from build123d import *

# Parameters (mm, degrees)
SKETCH1_W           = 76.2
SKETCH1_H           = 200.35
SKETCH1_R           = 19.05
SKETCH1_R_2         = 4.5
SKETCH1_R_3         = 3.25
BOSS_EXTRUDE1_DEPTH = 6.35


with BuildPart() as part:
    # Sketch1 → Boss-Extrude1 (new body)
    with BuildSketch(Plane.XY):
        with Locations((0, -25.175)):
            Rectangle(SKETCH1_W, SKETCH1_H)
        Circle(SKETCH1_R, mode=Mode.SUBTRACT)
        with Locations((0, 58.34)):
            Circle(SKETCH1_R_2, mode=Mode.SUBTRACT)
        with Locations((0, -58.34)):
            Circle(SKETCH1_R_2, mode=Mode.SUBTRACT)
        with Locations((-20, -110.35)):
            Circle(SKETCH1_R_3, mode=Mode.SUBTRACT)
        with Locations((20, -110.35)):
            Circle(SKETCH1_R_3, mode=Mode.SUBTRACT)
        with Locations((0, -77.35)):
            Circle(SKETCH1_R_3, mode=Mode.SUBTRACT)
    extrude(amount=BOSS_EXTRUDE1_DEPTH)


solid = part.part
Geometry: final body of the model. Coordinates: model frame, mm. Coordinates: 2 decimals unless noted, no trailing zeros. Loops run counter-clockwise (first coordinate to the right, second up) from the corner with the lowest first, then second, coordinate; pieces in that order, holes last. Notation, with made-up numbers: (71, -2.5) - (116, -2.5) arc R20 cw to (116, 29.5) - close; hole circle Ø6 at (62, 70). An arc over 180 degrees is marked (long way). One line per question, with ' | ' between items. Start each with the question number.
(1) Cut plane C-C on z = 3.25. Output: boundary loops of the cut face in (x, y).
(2) Ray query, L1, parallel to Y at x = 0, z = 4.5; L2, parallel to Y at x = -19.5, z = 1.75; L3, parallel to Y at x = 4, z = 3.5. Return the intervals inside material, ascending. Write a range as from..to.
(3) Cut plane B-B on x = 0. Output: boundary loops of the cut face in (y, z), and give its area (3 significant figures).
(4) Cut plane D-D on y = -110.35. Output: boundary loops of the cut face in (x, z).
(5) Draft query along Y for faces 1 (the flat face through (-1, -24, 6.35)), 2 (the cylindrical face through (-15.12, -11.59, 3.13)), 3 (the flat face through (-1, -125.35, 3)). Return one class per face: +Y half, -Y half, draft (parallel to the pull), parting line (faces both ways), or undercut.
(6) Cut plane A-A on y = -77.35. Output: boundary loops of the cut face in (x, z).
Here are the results:
1) outline: (-38.1, -125.35) - (38.1, -125.35) - (38.1, 75) - (-38.1, 75) - close; hole circle Ø6.5 at (-20, -110.35); hole circle Ø38.1 at (0, 0); hole circle Ø9 at (0, -58.34); hole circle Ø9 at (0, 58.34); hole circle Ø6.5 at (0, -77.35); hole circle Ø6.5 at (20, -110.35)
2) L1: -125.35..-80.6, -74.1..-62.84, -53.84..-19.05, 19.05..53.84, 62.84..75 | L2: -125.35..-113.56, -107.14..75 | L3: -125.35..-60.4, -56.28..-18.63, 18.63..56.28, 60.4..75
3) outline: (-125.35, 0) - (-80.6, 0) - (-80.6, 6.35) - (-125.35, 6.35) - close; (-74.1, 0) - (-62.84, 0) - (-62.84, 6.35) - (-74.1, 6.35) - close; (-53.84, 0) - (-19.05, 0) - (-19.05, 6.35) - (-53.84, 6.35) - close; (19.05, 0) - (53.84, 0) - (53.84, 6.35) - (19.05, 6.35) - close; (62.84, 0) - (75, 0) - (75, 6.35) - (62.84, 6.35) - close | area: 875 mm²
4) outline: (-38.1, 0) - (-23.25, 0) - (-23.25, 6.35) - (-38.1, 6.35) - close; (-16.75, 0) - (16.75, 0) - (16.75, 6.35) - (-16.75, 6.35) - close; (23.25, 0) - (38.1, 0) - (38.1, 6.35) - (23.25, 6.35) - close
5) face 1: draft | face 2: undercut | face 3: -Y half
6) outline: (-38.1, 0) - (-3.25, 0) - (-3.25, 6.35) - (-38.1, 6.35) - close; (3.25, 0) - (38.1, 0) - (38.1, 6.35) - (3.25, 6.35) - close
